```python
from build123d import *

# Parameters (mm, degrees)
SKETCH1_W                = 60.75
SKETCH1_H                = 11
SKETCH2_R                = 28.485
BOSS_EXTRUDE1_DEPTH      = 6.35
SKETCH3_W                = 6.475
SKETCH3_H                = 4.65
SKETCH4_W                = 6.475
SKETCH4_H                = 4.65
SKETCH5_W                = 6.475
SKETCH5_H                = 4.65
SKETCH6_W                = 6.475
SKETCH6_H                = 4.65
HOLE1_D                  = 5.1054
HOLE1_DEPTH              = 17.35
M8_CLEARANCE_HOLE1_D     = 9.8044
M8_CLEARANCE_HOLE1_DEPTH = 17.35
M45_CLEARANCE_HOLE1_D    = 49.911
M8_CLEARANCE_HOLE2_D     = 9.8044
CHAMFER1_SIZE            = 0.25
CHAMFER2_SIZE            = 1
CHAMFER3_SIZE            = 1.5


with BuildPart() as part:
    # Sketch1 → Revolve1 (revolve)
    with BuildSketch(Plane.XY, mode=Mode.PRIVATE) as revolve1_sk:
        with Locations((30.375, 5.5)):
            Rectangle(SKETCH1_W, SKETCH1_H)
    revolve(revolve1_sk.sketch.rotate(Axis((0, 11, 0), (0, -1, 0)), 270), axis=Axis((0, 11, 0), (0, -1, 0)))

    # Sketch2 → Boss-Extrude1 (add)
    with BuildSketch(Plane.XZ):
        with Locations(Location((0, 0, 0), (0, 0, 270))):
            Circle(SKETCH2_R)
    extrude(amount=BOSS_EXTRUDE1_DEPTH)

    # Sketch3 → Revolve2 (revolve)
    with BuildSketch(Plane(origin=(0, 0, 0), x_dir=(-1, 0, 0), z_dir=(0, 0, -1)), mode=Mode.PRIVATE) as revolve2_sk:
        with Locations((46.7625, -2.325)):
            Rectangle(SKETCH3_W, SKETCH3_H)
    revolve(revolve2_sk.sketch.rotate(Axis((-50, -4.65, 0), (0, 1, 0)), 270), axis=Axis((-50, -4.65, 0), (0, 1, 0)))

    # Sketch4 → Revolve3 (revolve)
    with BuildSketch(Plane(origin=(0, 0, -50), x_dir=(-1, 0, 0), z_dir=(0, 0, -1)), mode=Mode.PRIVATE) as revolve3_sk:
        with Locations((-3.2375, -2.325)):
            Rectangle(SKETCH4_W, SKETCH4_H)
    revolve(revolve3_sk.sketch.rotate(Axis((0, -4.65, -50), (0, 1, 0)), 270), axis=Axis((0, -4.65, -50), (0, 1, 0)))

    # Sketch5 → Revolve4 (revolve)
    with BuildSketch(Plane(origin=(0, 0, 0), x_dir=(-1, 0, 0), z_dir=(0, 0, -1)), mode=Mode.PRIVATE) as revolve4_sk:
        with Locations((-53.2375, -2.325)):
            Rectangle(SKETCH5_W, SKETCH5_H)
    revolve(revolve4_sk.sketch.rotate(Axis((50, -4.65, 0), (0, 1, 0)), 270), axis=Axis((50, -4.65, 0), (0, 1, 0)))

    # Sketch6 → Revolve5 (revolve)
    with BuildSketch(Plane(origin=(0, 0, 50), x_dir=(-1, 0, 0), z_dir=(0, 0, -1)), mode=Mode.PRIVATE) as revolve5_sk:
        with Locations((-3.2375, -2.325)):
            Rectangle(SKETCH6_W, SKETCH6_H)
    revolve(revolve5_sk.sketch.rotate(Axis((0, -4.65, 50), (0, 1, 0)), 270), axis=Axis((0, -4.65, 50), (0, 1, 0)))

    # Hole1
    with Locations(Plane(origin=(0, 11, 0), x_dir=(1, 0, 0), z_dir=(0, 1, 0))):
        with Locations((-34.648232278, -34.648232278), (34.648232278, -34.648232278), (34.648232278, 34.648232278), (-34.648232278, 34.648232278)):
            Hole(HOLE1_D / 2, depth=HOLE1_DEPTH)

    # M8 Clearance Hole1
    with Locations(Plane(origin=(0, 11, 0), x_dir=(1, 0, 0), z_dir=(0, 1, 0))):
        with Locations((50, 0), (0, -50), (-50, 0)):
            Hole(M8_CLEARANCE_HOLE1_D / 2, depth=M8_CLEARANCE_HOLE1_DEPTH)

    # M45 Clearance Hole1 (through all)
    with Locations(Plane(origin=(0, 11, 0), x_dir=(1, 0, 0), z_dir=(0, 1, 0))):
        with Locations((0, 0)):
            Hole(M45_CLEARANCE_HOLE1_D / 2)

    # M8 Clearance Hole2 (through all)
    with Locations(Plane(origin=(0, -4.65, 0), x_dir=(-1, 0, 0), z_dir=(0, -1, 0))):
        with Locations((0, 50)):
            Hole(M8_CLEARANCE_HOLE2_D / 2)

    # Chamfer1
    chamfer1_edges = [part.edges().sort_by_distance(p)[0] for p in [
        (-50, -4.65, -6.475),
        (0, -4.65, -56.475),
        (50, -4.65, -6.475),
        (0, -4.65, 43.525),
        (-45.0978, -4.65, 0),
        (4.9022, -4.65, 50),
        (54.9022, -4.65, 0),
        (24.9555, -6.35, 0),
        (-4.9022, -4.65, -50),
    ]]
    chamfer(chamfer1_edges, length=CHAMFER1_SIZE)

    # Chamfer2
    chamfer2_edges = [part.edges().sort_by_distance(p)[0] for p in [
        (0, -6.35, 28.485),
        (0, 0, 60.75),
        (0, 11, 60.75),
    ]]
    chamfer(chamfer2_edges, length=CHAMFER2_SIZE)

    # Chamfer3
    chamfer3_edges = [part.edges().sort_by_distance(p)[0] for p in [
        (-45.0978, 11, 0),
        (4.9022, 11, 50),
        (54.9022, 11, 0),
        (24.9555, 11, 0),
        (-4.9022, 11, -50),
    ]]
    chamfer(chamfer3_edges, length=CHAMFER3_SIZE)


solid = part.part
```
Verification items for the finished model (mm, model axes). A direction names the side the tool comes from. Round coordinates to 2 decimals unless told otherwise and drop trailing zeros.
1. Section check A-A on y = 5.25. State how many separate pieces and enclosed holes the cut face has, plus the area to 3 significant figures.
2. Draft check along Z on faces 1 (the cylindrical face through (-45.1, 2.5, -0.2)), 2 (the flat face through (-22.3, -6.35, -12.1)), 3 (the cylindrical face through (-59.3, 5.6, 13.2)). Enter one of: +Z half, -Z half, draft (parallel to the pull), parting line (faces both ways), or undercut.
3. Gauge pin test, flat ends, axial feed: P1, Ø4, axis at x = -12.5, y = 0, coming from the +Z side; P2, Ø15.5, axis at x = 50, z = 0, coming from the -Y side; P3, Ø6, axis at x = 1, z = -39.5, coming from the -Y side; P4, Ø4, axis at x = 34.65, z = 34.65, coming from the +Y side. Record the tip position at first contact, or that the pin passes through.
4. Scan lines: L1, parallel to X at y = 5, z = 0; L2, parallel to Z at x = -4, y = -3.5; L3, parallel to X at y = 4.5, z = 1.5. Record each from-to range of solid material in increasing order.
5. Access from +Z, -Z, +X, -X, +Y, -Y to the whole of each face (thin tool, end or side, straight path). Record for faces 4 (the cylindrical face through (-43.58, -2.17, -0.84)), 5 (the cylindrical face through (-34.32, 5.42, -37.18)), 6 (the flat face through (55, -4.65, -2)).
Answer:
1. separate pieces: 1
1. enclosed holes: 9
1. area: 9,250 mm2
2. face 1: undercut
2. face 2: draft
2. face 3: parting line
3. P1: stops at z = 59.79
3. P2: stops at y = -4.65
3. P3: stops at y = 0
3. P4: passes through
4. L1: x = -60.75 to -54.9, -45.1 to -24.96, 24.96 to 45.1, 54.9 to 60.75
4. L2: z = -55.09 to -52.83, -47.17 to -44.91, -28.2 to -24.63, 24.63 to 28.2, 44.91 to 47.17, 52.83 to 55.09
4. L3: x = -60.73 to -54.67, -45.33 to -24.91, 24.91 to 45.33, 54.67 to 60.73
5. face 4: -Y
5. face 5: +Y, -Y
5. face 6: +Z, -Z, +X, -Y
